Input: part model. Units: mm. Frame: model coordinates. Round coordinates to 2 decimals unless told otherwise and drop trailing zeros. Order: outer loops, then holes, each group sorted by start corner. A loop starts at its lowest first (then second) coordinate and runs counter-clockwise, first axis right, second up. Notation, with made-up numbers: (28.5, -27.75) -> (83.5, -27.75) arc R33 cw to (83.5, 4.25) -> close; hole circle Ø10 at (7, 2). An arc over 180 degrees is marked (long way). Use a Markdown table: item, result.
from build123d import *

# Parameters (mm, degrees)
SKETCH1_W           = 55
SKETCH1_H           = 55
BOSS_EXTRUDE1_DEPTH = 3
SKETCH2_W           = 10
SKETCH2_H           = 3
SKETCH2_W_2         = 15
CUT_EXTRUDE1_DEPTH  = 3
SKETCH3_W           = 55
SKETCH3_H           = 30
BOSS_EXTRUDE2_DEPTH = 3
SKETCH4_W           = 144
SKETCH4_H           = 52
BOSS_EXTRUDE3_DEPTH = 3
SKETCH5_W           = 199
SKETCH5_H           = 13
BOSS_EXTRUDE4_DEPTH = 3
SKETCH6_W           = 199
SKETCH6_H           = 20
BOSS_EXTRUDE5_DEPTH = 3
SKETCH7_R           = 2
SKETCH7_W           = 40
SKETCH7_H           = 20
CUT_EXTRUDE22_DEPTH = 33
SKETCH8_W           = 40
SKETCH8_H           = 9
CUT_EXTRUDE23_DEPTH = 33


with BuildPart() as part:
    # Sketch1 → Boss-Extrude1 (new body)
    with BuildSketch(Plane.XY):
        Rectangle(SKETCH1_W, SKETCH1_H)
    extrude(amount=BOSS_EXTRUDE1_DEPTH)

    # Sketch2 → Cut-Extrude1 (cut)
    with BuildSketch(Plane.XY.offset(3)):
        with Locations((22.5, -26)):
            Rectangle(SKETCH2_W, SKETCH2_H)
        with Locations((2.5, -26)):
            Rectangle(SKETCH2_W, SKETCH2_H)
        with Locations((-20, -26)):
            Rectangle(SKETCH2_W_2, SKETCH2_H)
    extrude(amount=-CUT_EXTRUDE1_DEPTH, mode=Mode.SUBTRACT)

    # Sketch3 → Boss-Extrude2 (add)
    with BuildSketch(Plane(origin=(0, 0, 0), x_dir=(-1, 0, 0), z_dir=(0, 0, -1))):
        with Locations((0, -42.5)):
            Rectangle(SKETCH3_W, SKETCH3_H)
    extrude(amount=-BOSS_EXTRUDE2_DEPTH)

    # Sketch4 → Boss-Extrude3 (add)
    with BuildSketch(Plane(origin=(0, 0, 0), x_dir=(-1, 0, 0), z_dir=(0, 0, -1))):
        with Locations((99.5, 1.5)):
            Rectangle(SKETCH4_W, SKETCH4_H)
    extrude(amount=-BOSS_EXTRUDE3_DEPTH)

    # Sketch5 → Boss-Extrude4 (add)
    with BuildSketch(Plane(origin=(0, 0, 0), x_dir=(-1, 0, 0), z_dir=(0, 0, -1))):
        with Locations((72, 34)):
            Rectangle(SKETCH5_W, SKETCH5_H)
    extrude(amount=-BOSS_EXTRUDE4_DEPTH)

    # Sketch6 → Boss-Extrude5 (add)
    with BuildSketch(Plane(origin=(0, 0, 0), x_dir=(-1, 0, 0), z_dir=(0, 0, -1))):
        with Locations((72, 50.5)):
            Rectangle(SKETCH6_W, SKETCH6_H)
    extrude(amount=-BOSS_EXTRUDE5_DEPTH)

    # Sketch7 → Cut-Extrude22 (cut)
    with BuildSketch(Plane(origin=(0, 0, 0), x_dir=(-1, 0, 0), z_dir=(0, 0, -1))):
        with Locations((168.5, 46.5)):
            Circle(SKETCH7_R)
        with Locations((168.5, 36.5)):
            Circle(SKETCH7_R)
        with Locations((118.5, 36.5)):
            Circle(SKETCH7_R)
        with Locations((118.5, 46.5)):
            Circle(SKETCH7_R)
        with Locations((143.5, 41.5)):
            Rectangle(SKETCH7_W, SKETCH7_H)
    extrude(amount=-CUT_EXTRUDE22_DEPTH, mode=Mode.SUBTRACT)

    # Sketch8 → Cut-Extrude23 (cut)
    with BuildSketch(Plane(origin=(0, 0, 0), x_dir=(-1, 0, 0), z_dir=(0, 0, -1))):
        with Locations((143.5, 56)):
            Rectangle(SKETCH8_W, SKETCH8_H)
    extrude(amount=-CUT_EXTRUDE23_DEPTH, mode=Mode.SUBTRACT)


solid = part.part
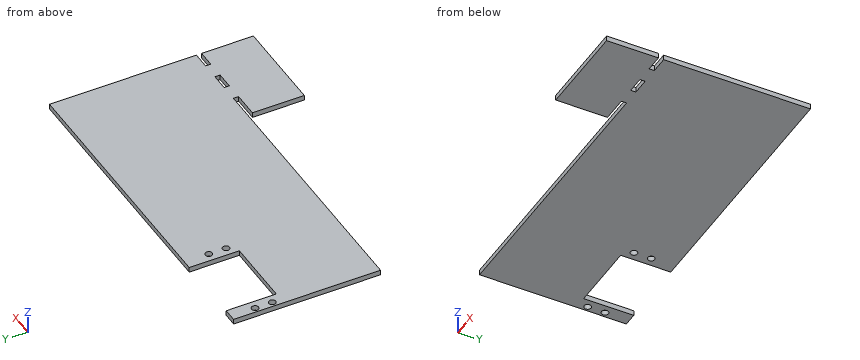
1) Pin query (flat end, axial travel): pin 1 Ø0.9 at (y, z) = (-26, 2) entering from -X; pin 2 Ø0.9 at (y, z) = (-47, 1.5) entering from -X; pin 3 Ø0.9 at (y, z) = (-25.5, 2) entering from +X. Return the tip coordinate at first contact, or that it passes through.
Results found:
| item | result |
|---|---|
| pin 1 | stops at x = -12.5 |
| pin 2 | stops at x = -27.5 |
| pin 3 | stops at x = 17.5 |
2) Cut plane C-C on z = 2.2. Return loops of the section in (x, y).
Results found:
| item | result |
|---|---|
| outline | (-171.5, -24.5) -> (-12.5, -24.5) -> (-12.5, -27.5) -> (-27.5, -27.5) -> (-27.5, -57.5) -> (27.5, -57.5) -> (27.5, -27.5) -> (17.5, -27.5) -> (17.5, -24.5) -> (27.5, -24.5) -> (27.5, 60.5) -> (-123.5, 60.5) -> (-123.5, 31.5) -> (-163.5, 31.5) -> (-163.5, 60.5) -> (-171.5, 60.5) -> close; hole circle Ø4 at (-168.5, 36.5); hole circle Ø4 at (-168.5, 46.5); hole circle Ø4 at (-118.5, 36.5); hole circle Ø4 at (-118.5, 46.5); hole (-2.5, -27.5) -> (7.5, -27.5) -> (7.5, -24.5) -> (-2.5, -24.5) -> close |
3) Cut plane D-D on y = -49. Return loops of the section in (x, z), and give its area (3 significant figures).
Results found:
| item | result |
|---|---|
| outline | (-27.5, 0) -> (27.5, 0) -> (27.5, 3) -> (-27.5, 3) -> close |
| area | 165 mm² |
4) Cut plane B-B on x = -118.5. Return loops of the section in (y, z).
Results found:
| item | result |
|---|---|
| outline | (-24.5, 0) -> (34.5, 0) -> (34.5, 3) -> (-24.5, 3) -> close; (38.5, 0) -> (44.5, 0) -> (44.5, 3) -> (38.5, 3) -> close; (48.5, 0) -> (60.5, 0) -> (60.5, 3) -> (48.5, 3) -> close |
5) Line query: L1, parallel to Y at x = -168.5, z = 1.25; L2, parallel to Y at x = -19, z = 1.7; L3, parallel to Y at x = -95.5, z = 2.6. Output: solid intervals per line, ascending. Write a range as [from, to].
Results found:
| item | result |
|---|---|
| L1 | y = [-24.5, 34.5], [38.5, 44.5], [48.5, 60.5] |
| L2 | y = [-57.5, -27.5], [-24.5, 60.5] |
| L3 | y = [-24.5, 60.5] |
6) Cut plane A-A on y = 36.5. Return loops of the section in (x, z), and give its area (3 significant figures).
Results found:
| item | result |
|---|---|
| outline | (-171.5, 0) -> (-170.5, 0) -> (-170.5, 3) -> (-171.5, 3) -> close; (-166.5, 0) -> (-163.5, 0) -> (-163.5, 3) -> (-166.5, 3) -> close; (-123.5, 0) -> (-120.5, 0) -> (-120.5, 3) -> (-123.5, 3) -> close; (-116.5, 0) -> (27.5, 0) -> (27.5, 3) -> (-116.5, 3) -> close |
| area | 453 mm² |
